For this review, take the finished solid that the model builds, in its own axes (mm). Round coordinates to 2 decimals unless told otherwise and drop trailing zeros. Order: outer loops, then holes, each group sorted by start corner. A loop starts at its lowest first (then second) coordinate and runs counter-clockwise, first axis right, second up.
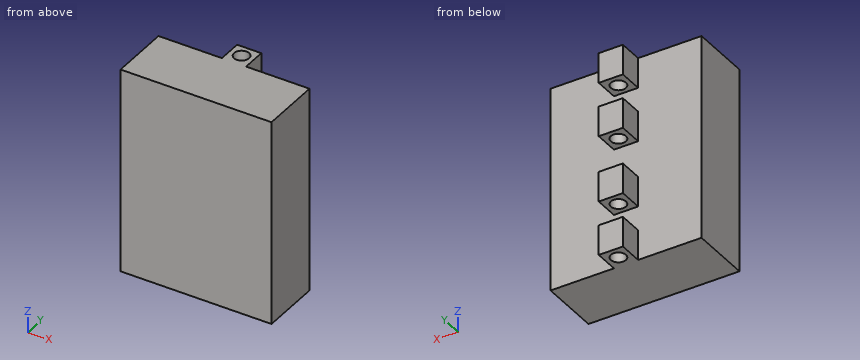
```python
from build123d import *

# Parameters (mm, degrees)
SKETCH1_W           = 250
SKETCH1_H           = 340
BOSS_EXTRUDE1_DEPTH = 100
SKETCH3_R           = 12.5
BOSS_EXTRUDE2_DEPTH = 340
SKETCH4_W           = 40
SKETCH4_H           = 40
SKETCH4_H_2         = 60
CUT_EXTRUDE1_DEPTH  = 40


with BuildPart() as part:
    # Sketch1 → Boss-Extrude1 (new body)
    with BuildSketch(Plane(origin=(0, 0, 0), x_dir=(1, 0, 0), z_dir=(0, 1, 0))):
        with Locations((125, -170)):
            Rectangle(SKETCH1_W, SKETCH1_H)
    extrude(amount=BOSS_EXTRUDE1_DEPTH)

    # Sketch3 → Boss-Extrude2 (add, through all)
    with BuildSketch(Plane.XY.offset(340)):
        Polygon((105, 100), (145, 100), (145, 120), (145, 132.5), (145, 140), (105, 140), (105, 132.5), (105, 120), align=None)
        with Locations((125, 120)):
            Circle(SKETCH3_R, mode=Mode.SUBTRACT)
    extrude(amount=-BOSS_EXTRUDE2_DEPTH)

    # Sketch4 → Cut-Extrude1 (cut)
    with BuildSketch(Plane(origin=(0, 140, 0), x_dir=(1, 0, 0), z_dir=(0, 1, 0))):
        with Locations((125, -270)):
            Rectangle(SKETCH4_W, SKETCH4_H)
        with Locations((125, -70)):
            Rectangle(SKETCH4_W, SKETCH4_H)
        with Locations((125, -170)):
            Rectangle(SKETCH4_W, SKETCH4_H_2)
    extrude(amount=-CUT_EXTRUDE1_DEPTH, mode=Mode.SUBTRACT)


solid = part.part
```
Q1. Take a section at A-A, the plane x = 125. Count the separate pieces of the cut face and the enclosed holes in it, plus the area to 3 significant figures.
Q2. Take a section at D-D, the plane x = 100. State the section outline as (y, z) points, plus the area to 3 significant figures.
Q3. Take a section at C-C, the plane z = 296. State the section outline as (x, y) points, plus the area to 3 significant figures.
Q4. Wall thickness on line 1 (Z direction, x = 136, y = 127); line 2 (Y direction, x = 125, z = 216); line 3 (Y direction, x = 50.5, z = 197.5): over which ranges is each line inside the solid? List them lowest first.
Q5. Clearance check with flat-ended pins moving along their axes: pin 1 (20 mm diameter, centred on y = 130, z = 116, fed in from +X); pin 2 (8 mm diameter, centred on x = 59.5, z = 264.5, fed in from +Y); pin 3 (12 mm diameter, centred on y = 116, z = 227.5, fed in from -X); pin 4 (12 mm diameter, centred on x = 124.5, y = 117.5, fed in from +Z). State where each tip first meets the part, or that it passes through.
Working result:
1. separate pieces: 5
1. enclosed holes: 0
1. area: 37,000 mm2
2. outline: (0, 0) - (100, 0) - (100, 340) - (0, 340) - close
2. area: 34,000 mm2
3. outline: (0, 0) - (250, 0) - (250, 100) - (145, 100) - (145, 140) - (105, 140) - (105, 100) - (0, 100) - close; hole circle Ø25 at (125, 120)
3. area: 26,100 mm2
4. line 1: z = 0 to 50, 90 to 140, 200 to 250, 290 to 340
4. line 2: y = 0 to 107.5, 132.5 to 140
4. line 3: y = 0 to 100
5. pin 1: stops at x = 145
5. pin 2: stops at y = 100
5. pin 3: stops at x = 105
5. pin 4: passes through
